Part print with two shaded views. Sizes in mm from the minimum x, y, z corner. A direction names the side the tool comes from. Round coordinates to 2 decimals unless told otherwise and drop trailing zeros. Write each loop counter-clockwise with the first axis right and the second up, starting at its lowest first coordinate (ties: lowest second). Pieces come first, ordered by that corner, then holes. Notation, with made-up numbers: (41, 0.5) -> (48, 0.5) arc R15 cw to (48, 6.5) -> close; hole circle Ø10 at (22, -30.5). An arc over 180 degrees is marked (long way). Put each result on its own line as item: value. Start each with the question number.
1. Pull direction X, two halves, no side cores. Call the marked faces 4, 5 and 6: pulls with the +X half, pulls with the -X half, needs draft (parallel to the pull), parting line crosses it, or undercut.
2. Flat gauge pins, fed straight in: P1, Ø2, axis at y = 20, z = 46, coming from the -X side (1 decimal); P2, Ø2, axis at x = 20, y = 19, coming from the +Z side; P3, Ø11.5, axis at x = 41.5, z = 55, coming from the +Y side (3 decimals). Where does each tip first touch, or does it go through?
3. Drill centre lines: line 1 (Y direction, x = 31.5, z = 52) (1 decimal); line 2 (X direction, y = 2.75, z = 15); line 3 (Y direction, x = 80.5, z = 18) (1 decimal). Where is each one in solid material? Low to high. Write a range as from..to.
4. Saw through at A-A on y = 20.5. List the corners of the cut face in (x, z) (1 decimal).
5. 3-axis set-ups, long thin cutter, end or side, ignore diameter. For the marked faces 1, 2 and 3: which of +Z, -Z, +X, -X, +Y, -Y reach the whole face in a straight line?
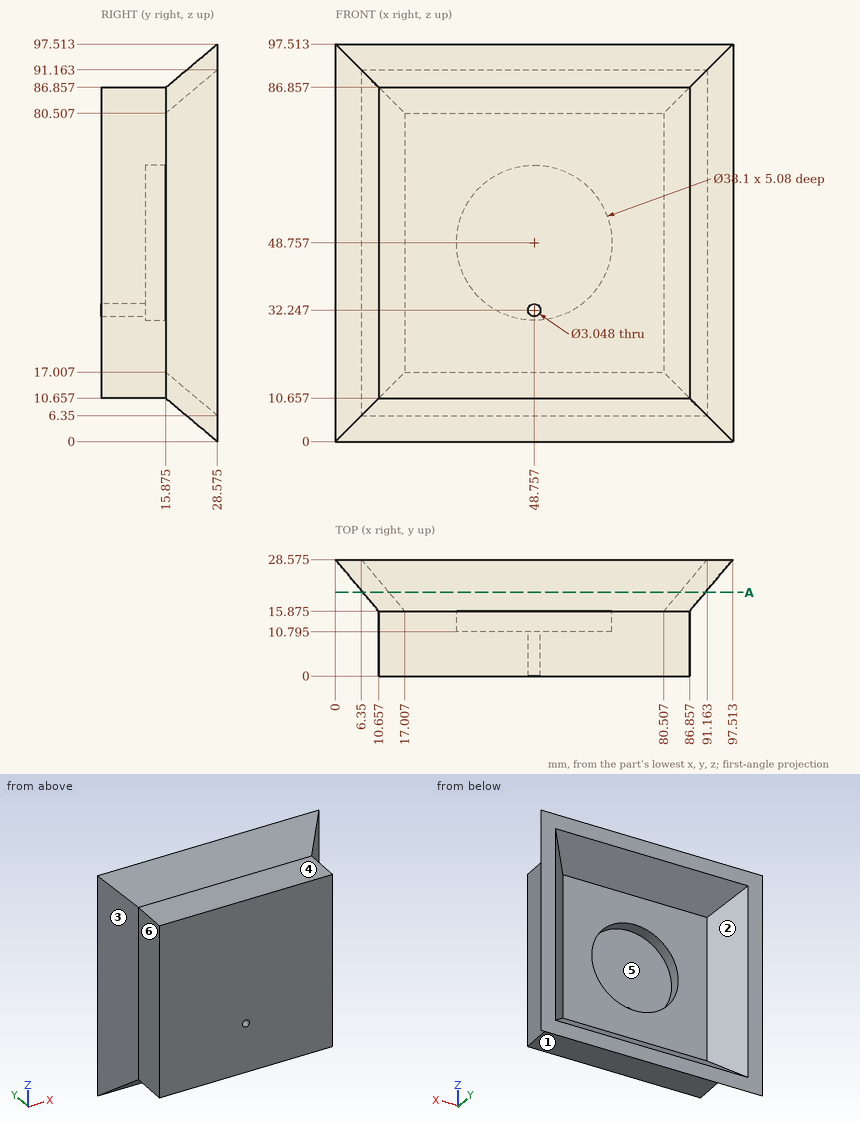
Return value:
1. face 4: needs draft
1. face 5: undercut
1. face 6: pulls with the -X half
2. P1: stops at x = 6.4
2. P2: stops at z = 90.32
2. P3: stops at y = 10.795
3. line 1: y = 0..10.8
3. line 2: x = 10.66..86.86
3. line 3: y = 0..15.9
4. outline: (6.8, 6.8) -> (90.7, 6.8) -> (90.7, 90.7) -> (6.8, 90.7) -> close; hole (13.1, 13.1) -> (84.4, 13.1) -> (84.4, 84.4) -> (13.1, 84.4) -> close
5. face 1: -Z, +X, -X, -Y
5. face 2: +Y
5. face 3: +Z, -Z, -X, -Y
